Autodesk Inventor part; units mm, degrees
sketch "Skizze1" plane through (0, 0, 0) normal (0, 0, 1) x (1, 0, 0)
  circle A0 centre (0, 0) radius 5
  line L0 (0, 81.3997) -> (0, -19.4)
  circle A1 centre (0, 0) radius 4.25
  point P0 (37.012, 66.9998)
  dimension "d0" = 10
  dimension "d1" = 8.5
extrude "Extrusion1" add sketch "Skizze1" along normal mid plane 10 contours A0 L0 A1 | L0 A1 A0
sketch "Skizze2" plane through (0, 0, 5) normal (0, 0, 1) x (1, 0, 0)
  circle A0 centre (0, 0) radius 5
extrude "Extrusion2" add sketch "Skizze2" against normal blind 2
fillet "Rundung1" radius 2 1 edges at (-4.25, 0, 3)
fillet "Rundung2" radius 2 1 edges at (-5, 0, 5)
properties part number "Sirene"
Read the model definition and answer for the solid it produces. Units are mm, in the model's axes. A direction names the side the tool comes from. Give positions to 0.01 mm unless a question says otherwise; leave off trailing zeros. Write each loop counter-clockwise with the first axis right and the second up, starting at its lowest first coordinate (ties: lowest second). Pieces come first, ordered by that corner, then holes. Notation, with made-up numbers: (-16.5, 86) -> (23.5, 86) arc R22 ccw to (23.5, 106) -> close; hole circle Ø3 at (52, -26). An arc over 180 degrees is marked (long way). Answer as a JSON object with one key per item and string values. Group by question number.
1) The mould has two halves that part along X. Classify faces 3 (the cylindrical face through (2.285, 3.584, -1.958)), 4 (the cylindrical face through (-1.08, -4.88, -0.94)), 5 (the flat face through (-2, -4, -5)): +X half, -X half, draft (parallel to the pull), parting line (faces both ways), or undercut.
2) Each of these flat-tipped pins is pushed along its axis until it touches: P1, Ø2, axis at x = -4, z = -1.5, coming from the -Y side; P2, Ø1, axis at y = 1, z = -0.5, coming from the +X side; P3, Ø3, axis at y = -1.5, z = -3.5, coming from the -X side; P4, Ø1.5, axis at x = -4, y = 3, coming from the +Z side. Where does it stop, or does it pass through?
3) Find section C-C (z = -3). Write down the section's boundary in (x, y).
4) Find section A-A (y = 0). Write down the section's boundary in (x, z), and give its area (3 significant figures).
5) Consider L1, parallel to X at y = 0, z = -1.9; L2, parallel to Y at x = 2, z = 2. Determine where each line is inside the solid, lowest interval first. Write a range as from..to.
6) A tool of negligible diameter and unlimited length cuts with its end or side. For faces 1 (the flat face through (0, 0, 5)), 2 (the flat face through (0, 0, 3)), from which of +Z, -Z, +X, -X, +Y, -Y can it reach the whole face along a straight path? Write none if from no direction.
Values follow:
{
 "1": {"face 3": "undercut", "face 4": "parting line", "face 5": "draft"},
 "2": {"P1": "stops at y = -4", "P2": "stops at x = 4.97", "P3": "stops at x = -5", "P4": "stops at z = 4.56"},
 "3": {"outline": "circle Ø10 at (0, 0); hole circle Ø8.5 at (0, 0)"},
 "4": {"outline": "(-5, -5) -> (-4.25, -5) -> (-4.25, 1) arc R2 cw to (-2.25, 3) -> (2.25, 3) arc R2 cw to (4.25, 1) -> (4.25, -5) -> (5, -5) -> (5, 3) arc R2 ccw to (3, 5) -> (-3, 5) arc R2 ccw to (-5, 3) -> close", "area": "32.0 mm2"},
 "5": {"L1": "x = -5..-4.25, 4.25..5", "L2": "y = -4.58..-3.44, 3.44..4.58"},
 "6": {"face 1": "+Z, +X, -X, +Y, -Y", "face 2": "-Z"}
}
